Check sheet for the modelled part. Datum: model origin and axes. Units: mm. Face numbers are marked on the shaded views. A direction names the side the tool comes from. Give positions to 0.01 mm unless a question says otherwise; leave off trailing zeros. Order: outer loops, then holes, each group sorted by start corner. A loop starts at its lowest first (then second) coordinate and runs counter-clockwise, first axis right, second up. Notation, with made-up numbers: (73, 88.25) -> (88, 88.25) arc R17 cw to (88, 95.25) -> close; hole circle Ø9 at (-14, -5). An arc over 180 degrees is marked (long way). One line per question, with ' | ' between items. Start each with the question number.
from build123d import *

# Parameters (mm, degrees)
SKETCH1_R           = 49.2125
BASE_EXTRUDE_DEPTH  = 3.175
SKETCH5_R           = 3.175
CUT_EXTRUDE2_DEPTH  = 4.175
CIRPATTERN1_COUNT   = 4
SKETCH2_R           = 36.5125
BOSS_EXTRUDE1_DEPTH = 12.7
SKETCH3_R           = 12.7
BOSS_EXTRUDE2_DEPTH = 12.7
FILLET1_R           = 3.175
SKETCH6_W           = 5.08
SKETCH6_H           = 9.525
BOSS_EXTRUDE3_DEPTH = 47.625
SKETCH4_R           = 7.9375
CUT_EXTRUDE1_DEPTH  = 29.575
FILLET2_R           = 3.175
CUT_EXTRUDE3_REACH  = 53.752
SKETCH7_R           = 1.5875
FILLET3_R           = 1.5875


with BuildPart() as part:
    # Sketch1 → Base-Extrude (new body)
    with BuildSketch(Plane.XY):
        Circle(SKETCH1_R)
    extrude(amount=BASE_EXTRUDE_DEPTH)

    # Sketch5 → Cut-Extrude2 (cut, through all)
    with BuildSketch(Plane.XY.offset(3.175)):
        with Locations((31.430896424, 31.430896424)):
            Circle(SKETCH5_R)
    cut_extrude2 = extrude(amount=-CUT_EXTRUDE2_DEPTH, mode=Mode.SUBTRACT)

    # CirPattern1: Cut-Extrude2 ×4 about axis
    cirpattern1_axis = Axis((0, 0, 0), (0, 0, 1))
    for i in range(1, CIRPATTERN1_COUNT):
        add(cut_extrude2.rotate(cirpattern1_axis, i * 360 / CIRPATTERN1_COUNT), mode=Mode.SUBTRACT)

    # Sketch2 → Boss-Extrude1 (add)
    with BuildSketch(Plane.XY.offset(3.175)):
        Circle(SKETCH2_R)
    extrude(amount=BOSS_EXTRUDE1_DEPTH)

    # Sketch3 → Boss-Extrude2 (add)
    with BuildSketch(Plane.XY.offset(15.875)):
        Circle(SKETCH3_R)
    extrude(amount=BOSS_EXTRUDE2_DEPTH)

    # Fillet1
    fillet1_edges = [part.edges().sort_by_distance(p)[0] for p in [
        (-36.5125, 0, 3.175),
        (-12.7, 0, 15.875),
    ]]
    fillet(fillet1_edges, radius=FILLET1_R)

    # Sketch6 → Boss-Extrude3 (add)
    with BuildSketch(Plane(origin=(0, 0, 0), x_dir=(1, 0, 0), z_dir=(0, 1, 0))):
        with Locations((0, -7.9375)):
            Rectangle(SKETCH6_W, SKETCH6_H)
    extrude(amount=BOSS_EXTRUDE3_DEPTH)

    # Sketch4 → Cut-Extrude1 (cut, through all)
    with BuildSketch(Plane.XY.offset(28.575)):
        Circle(SKETCH4_R)
    extrude(amount=-CUT_EXTRUDE1_DEPTH, mode=Mode.SUBTRACT)

    # Fillet2
    fillet2_edges = [part.edges().sort_by_distance(p)[0] for p in [
        (0, 47.625, 12.7),
    ]]
    fillet(fillet2_edges, radius=FILLET2_R)

    # Sketch7 → Cut-Extrude3 (cut, up to next)
    with BuildSketch(Plane(origin=(2.54, 0, 0), x_dir=(0, 0, -1), z_dir=(1, 0, 0)), mode=Mode.PRIVATE) as cut_extrude3_sk1:
        with Locations((-9.525, 44.45)):
            Circle(SKETCH7_R)
    cut_extrude3_tool1 = extrude(cut_extrude3_sk1.sketch, amount=-CUT_EXTRUDE3_REACH, mode=Mode.PRIVATE) & part.part
    add(cut_extrude3_tool1.solids().sort_by_distance((2.54, 44.45, 9.525))[0], mode=Mode.SUBTRACT)

    # Fillet3
    fillet3_edges = [part.edges().sort_by_distance(p)[0] for p in [
        (-2.54, 36.424045029, 9.5249997),
        (-2.54, 43.615568299, 3.175),
        (2.54, 43.615568299, 3.175),
        (2.54, 36.424045029, 9.5249997),
    ]]
    fillet(fillet3_edges, radius=FILLET3_R)


solid = part.part
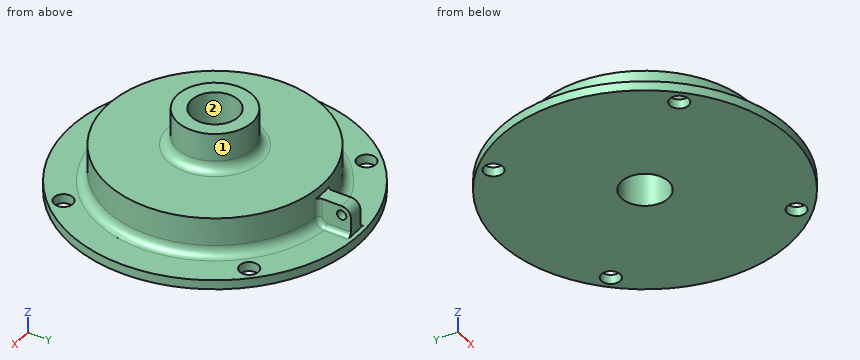
1. Tool access check on the marked faces 1 and 2. Record the directions out of +Z, -Z, +X, -X, +Y, -Y that give a thin tool (end or side, any length) a straight path to the whole face; none if there is none.
2. Cross-section at C-C on z = 25. Record the boundary of the cut face in (x, y) (1 decimal).
3. Cross-section at D-D on x = -41.5. Record the boundary of the cut face in (y, z) (3 decimals), and give its area (3 significant figures).
4. Scan lines: probe 1 along Y at (x, z) = (0, 6.25) (1 decimal); probe 2 along X at (y, z) = (40.5, 4.75); probe 3 along X at (y, z) = (-13, 4.75). Record each from-to range of solid material in increasing order.
5. Cross-section at A-A on x = 0. Give the number of separate pieces and of enclosed holes in the cut face, and give its area (3 significant figures).
6. Go/stop test with flat-tipped pins: pin 1 (10 mm diameter, centred on x = -31.43, y = 31.43, fed in from +Z); pin 2 (12.5 mm diameter, centred on x = 0, y = 0, fed in from -Z); pin 3 (5 mm diameter, centred on x = 4, y = 14.5, fed in from +Z) (3 decimals); pin 4 (2.5 mm diameter, centred on x = -1, y = 39.5, fed in from +Z). Record where each tip stops, or that it passes through.
Response values:
1) face 1: +Z | face 2: +Z, -Z
2) outline: circle Ø25.4 at (0, 0); hole circle Ø15.9 at (0, 0)
3) outline: (-26.45, 0) -> (26.45, 0) -> (26.45, 3.175) -> (-26.45, 3.175) -> close | area: 168 mm²
4) probe 1: y = -36.5 to -7.9, 7.9 to 47.6 | probe 2: x = -2.54 to 2.54 | probe 3: x = -34.58 to 34.58
5) separate pieces: 2 | enclosed holes: 1 | area: 1,210 mm²
6) pin 1: stops at z = 3.18 | pin 2: passes through | pin 3: stops at z = 28.575 | pin 4: stops at z = 12.7
